The listing builds one solid part. Answer for the finished solid, in the listing's coordinates (mm). Round coordinates to 2 decimals unless told otherwise and drop trailing zeros. Order: outer loops, then holes, each group sorted by start corner. A loop starts at its lowest first (then second) coordinate and runs counter-clockwise, first axis right, second up. Notation, with made-up numbers: M -20.75,-38 L -6.75,-38 A26 ccw -6.75,-8 Z; hole C 19,-25 d4. An arc over 180 degrees is marked long. Write item = value, one per line. Start each with the question number.
(1) Straight lines are drawn through the part: probe 1 along Y at (x, z) = (7.45, -2.75); probe 2 along X at (y, z) = (4.75, -3.75); probe 3 along X at (y, z) = (3, 0.5). For each, find the intervals that lie inside material, in ascending order. Write a range as from..to.
(2) A cutting plane is placed at D-D, the plane y = 5.75. Determine the outline of the cut face in (x, z) (3 decimals).
(3) This flat-tipped pin is pushed along its axis until it touches: pin 1 (1.8 mm diameter, centred on x = -15.98, z = -0.88, fed in from +Y) (3 decimals). Where does it stop, or does it pass through?
(4) A cutting plane is placed at B-B, the plane z = -1.5. Determine the outline of the cut face in (x, y).
(5) A cutting plane is placed at C-C, the plane x = 7.45. Determine the outline of the cut face in (y, z) (3 decimals), and give its area (3 significant figures).
(6) For a pull along Z with two mould halves and no side action, classify faces 1 (the face through (-0.3, 7.5, 4.875)), 2 (the face through (0, 8, 0)), 3 (the face through (14.49, 3.94, -0.68)) as released by +Z, released by -Z, zero draft, split by the parting line, or undercut.
(7) A cutting plane is placed at A-A, the plane y = 3.25. Determine the outline of the cut face in (x, z) (3 decimals), and give its area (3 significant figures).
from build123d import *

# Parameters (mm, degrees)
SKETCH1_W           = 40
SKETCH1_H           = 9.75
SKETCH1_R           = 1.5
BOSS_EXTRUDE1_DEPTH = 8
CUT_EXTRUDE1_REACH  = 25.645
CUT_EXTRUDE2_REACH  = 25.645
SKETCH3_R           = 1.4


with BuildPart() as part:
    # Sketch1 → Boss-Extrude1 (new body)
    with BuildSketch(Plane(origin=(0, 0, 0), x_dir=(1, 0, 0), z_dir=(0, 1, 0))):
        Rectangle(SKETCH1_W, SKETCH1_H)
        with Locations(Location((-15.976056303, 0.875, 0), (0, 0, 270))):
            Circle(SKETCH1_R, mode=Mode.SUBTRACT)
        with Locations(Location((15.976056303, 0.875, 0), (0, 0, 90))):
            Circle(SKETCH1_R, mode=Mode.SUBTRACT)
    extrude(amount=BOSS_EXTRUDE1_DEPTH)

    # Sketch2 → Cut-Extrude1 (cut, up to next)
    with BuildSketch(Plane.XY.offset(4.875), mode=Mode.PRIVATE) as cut_extrude1_sk1:
        with BuildLine():
            ThreePointArc((3, 4), (2.121320344, 6.121320344), (0, 7))
            Line((0, 7), (0, 1))
            ThreePointArc((0, 1), (2.121320344, 1.878679656), (3, 4))
        make_face()
    cut_extrude1_tool1 = extrude(cut_extrude1_sk1.sketch, amount=-CUT_EXTRUDE1_REACH, mode=Mode.PRIVATE) & part.part
    # Sketch2 → Cut-Extrude1 (cut, up to next)
    with BuildSketch(Plane.XY.offset(4.875), mode=Mode.PRIVATE) as cut_extrude1_sk2:
        with BuildLine():
            Line((0, 1), (0, 7))
            ThreePointArc((0, 7), (-3, 4), (0, 1))
        make_face()
    cut_extrude1_tool2 = extrude(cut_extrude1_sk2.sketch, amount=-CUT_EXTRUDE1_REACH, mode=Mode.PRIVATE) & part.part
    # Sketch2 → Cut-Extrude1 (cut, up to next)
    with BuildSketch(Plane.XY.offset(4.875), mode=Mode.PRIVATE) as cut_extrude1_sk3:
        with BuildLine():
            ThreePointArc((3, 4), (2.121320344, 6.121320344), (0, 7))
            Line((0, 7), (0, 1))
            ThreePointArc((0, 1), (2.121320344, 1.878679656), (3, 4))
        make_face()
    cut_extrude1_tool3 = extrude(cut_extrude1_sk3.sketch, amount=-CUT_EXTRUDE1_REACH, mode=Mode.PRIVATE) & part.part
    # Sketch2 → Cut-Extrude1 (cut, up to next)
    with BuildSketch(Plane.XY.offset(4.875), mode=Mode.PRIVATE) as cut_extrude1_sk4:
        with BuildLine():
            Line((0, 1), (0, 7))
            ThreePointArc((0, 7), (-3, 4), (0, 1))
        make_face()
    cut_extrude1_tool4 = extrude(cut_extrude1_sk4.sketch, amount=-CUT_EXTRUDE1_REACH, mode=Mode.PRIVATE) & part.part
    add(cut_extrude1_tool1.solids().sort_by_distance((1.27324, 4, 4.875))[0], mode=Mode.SUBTRACT)
    add(cut_extrude1_tool2.solids().sort_by_distance((-1.27324, 4, 4.875))[0], mode=Mode.SUBTRACT)
    add(cut_extrude1_tool3.solids().sort_by_distance((1.27324, 4, 4.875))[0], mode=Mode.SUBTRACT)
    add(cut_extrude1_tool4.solids().sort_by_distance((-1.27324, 4, 4.875))[0], mode=Mode.SUBTRACT)

    # Sketch3 → Cut-Extrude2 (cut, up to next)
    with BuildSketch(Plane(origin=(0, 0, -4.875), x_dir=(-1, 0, 0), z_dir=(0, 0, -1)), mode=Mode.PRIVATE) as cut_extrude2_sk1:
        with Locations((7.45, 4)):
            Circle(SKETCH3_R)
    cut_extrude2_tool1 = extrude(cut_extrude2_sk1.sketch, amount=-CUT_EXTRUDE2_REACH, mode=Mode.PRIVATE) & part.part
    # Sketch3 → Cut-Extrude2 (cut, up to next)
    with BuildSketch(Plane(origin=(0, 0, -4.875), x_dir=(-1, 0, 0), z_dir=(0, 0, -1)), mode=Mode.PRIVATE) as cut_extrude2_sk2:
        with Locations((-7.45, 4)):
            Circle(SKETCH3_R)
    cut_extrude2_tool2 = extrude(cut_extrude2_sk2.sketch, amount=-CUT_EXTRUDE2_REACH, mode=Mode.PRIVATE) & part.part
    add(cut_extrude2_tool1.solids().sort_by_distance((-7.45, 4, -4.875))[0], mode=Mode.SUBTRACT)
    add(cut_extrude2_tool2.solids().sort_by_distance((7.45, 4, -4.875))[0], mode=Mode.SUBTRACT)


solid = part.part
Reported:
q1.probe_1 = 0..2.6, 5.4..8
q1.probe_2 = -20..-8.63, -6.27..-2.9, 2.9..6.27, 8.63..20
q1.probe_3 = -20..-16.58, -15.38..-8.43, -6.47..-2.83, 2.83..6.47, 8.43..15.38, 16.58..20
q2.outline = M -20,-4.875 L -2.437,-4.875 L -2.437,4.875 L -20,4.875 Z; M 2.437,-4.875 L 20,-4.875 L 20,4.875 L 2.437,4.875 Z; hole C -15.976,-0.875 d3; hole C 15.976,-0.875 d3
q3.pin_1 = through
q4.outline = M -20,0 L -17.34,0 L -17.34,8 L -20,8 Z; M -14.61,0 L 14.61,0 L 14.61,8 L -14.61,8 Z; M 17.34,0 L 20,0 L 20,8 L 17.34,8 Z; hole C -7.45,4 d2.8; hole C 0,4 d6; hole C 7.45,4 d2.8
q5.outline = M 0,-4.875 L 2.6,-4.875 L 2.6,4.875 L 0,4.875 Z; M 5.4,-4.875 L 8,-4.875 L 8,4.875 L 5.4,4.875 Z
q5.area = 50.7 mm²
q6.face_1 = released by +Z
q6.face_2 = zero draft
q6.face_3 = undercut
q7.outline = M -20,-4.875 L -8.632,-4.875 L -8.632,4.875 L -20,4.875 Z; M -6.268,-4.875 L -2.905,-4.875 L -2.905,4.875 L -6.268,4.875 Z; M 2.905,-4.875 L 6.268,-4.875 L 6.268,4.875 L 2.905,4.875 Z; M 8.632,-4.875 L 20,-4.875 L 20,4.875 L 8.632,4.875 Z; hole C -15.976,-0.875 d3; hole C 15.976,-0.875 d3
q7.area = 273 mm²
